from build123d import *

# Parameters (mm, degrees)
SKETCH1_R           = 15
SKETCH1_R_2         = 1.25
SKETCH1_R_3         = 3
BOSS_EXTRUDE1_DEPTH = 5
SKETCH4_R           = 5.5
SKETCH4_R_2         = 5
CUT_EXTRUDE1_DEPTH  = 0.2
SKETCH4_3_R         = 5
SKETCH4_3_R_2       = 3.5
CUT_EXTRUDE2_DEPTH  = 0.1
CUT_EXTRUDE3_START  = -0.1
SKETCH5_R           = 5
SKETCH5_R_2         = 3.5
CUT_EXTRUDE3_DEPTH  = 0.1
CUT_EXTRUDE4_START  = -0.2
SKETCH5_3_R         = 5.75
SKETCH5_3_R_2       = 5
CUT_EXTRUDE4_DEPTH  = 0.2
FILLET1_R           = 0.1


with BuildPart() as part:
    # Sketch1 → Boss-Extrude1 (new body)
    with BuildSketch(Plane(origin=(0, 0, 0), x_dir=(1, 0, 0), z_dir=(0, 1, 0))):
        with Locations(Location((0, 0, 0), (0, 0, 270))):
            Circle(SKETCH1_R)
        with Locations(Location((0, 12, 0), (0, 0, 270))):
            Circle(SKETCH1_R_2, mode=Mode.SUBTRACT)
        with Locations(Location((0, -12, 0), (0, 0, 270))):
            Circle(SKETCH1_R_2, mode=Mode.SUBTRACT)
        with Locations(Location((0, 0, 0), (0, 0, 270))):
            Circle(SKETCH1_R_3, mode=Mode.SUBTRACT)
        with Locations(Location((-12, 0, 0), (0, 0, 270))):
            Circle(SKETCH1_R_2, mode=Mode.SUBTRACT)
        with Locations(Location((12, 0, 0), (0, 0, 270))):
            Circle(SKETCH1_R_2, mode=Mode.SUBTRACT)
        with Locations(Location((8.5, 8.5, 0), (0, 0, 270))):
            Circle(SKETCH1_R_2, mode=Mode.SUBTRACT)
        with Locations(Location((8.5, -8.5, 0), (0, 0, 270))):
            Circle(SKETCH1_R_2, mode=Mode.SUBTRACT)
        with Locations(Location((-8.5, -8.5, 0), (0, 0, 270))):
            Circle(SKETCH1_R_2, mode=Mode.SUBTRACT)
        with Locations(Location((-8.5, 8.5, 0), (0, 0, 270))):
            Circle(SKETCH1_R_2, mode=Mode.SUBTRACT)
    extrude(amount=BOSS_EXTRUDE1_DEPTH)

    # Sketch4 → Cut-Extrude1 (cut)
    with BuildSketch(Plane(origin=(0, 5, 0), x_dir=(1, 0, 0), z_dir=(0, 1, 0))):
        with Locations(Location((0, 0, 0), (0, 0, 270))):
            Circle(SKETCH4_R)
        with Locations(Location((0, 0, 0), (0, 0, 270))):
            Circle(SKETCH4_R_2, mode=Mode.SUBTRACT)
    extrude(amount=-CUT_EXTRUDE1_DEPTH, mode=Mode.SUBTRACT)

    # Sketch4<3> → Cut-Extrude2 (cut)
    with BuildSketch(Plane(origin=(0, 5, 0), x_dir=(1, 0, 0), z_dir=(0, 1, 0))):
        with Locations(Location((0, 0, 0), (0, 0, 270))):
            Circle(SKETCH4_3_R)
        with Locations(Location((0, 0, 0), (0, 0, 270))):
            Circle(SKETCH4_3_R_2, mode=Mode.SUBTRACT)
    extrude(amount=-CUT_EXTRUDE2_DEPTH, mode=Mode.SUBTRACT)

    # Sketch5 → Cut-Extrude3 (cut)
    with BuildSketch(Plane.XZ.offset(CUT_EXTRUDE3_START)):
        with Locations(Location((0, 0, 0), (0, 0, 90))):
            Circle(SKETCH5_R)
        with Locations(Location((0, 0, 0), (0, 0, 90))):
            Circle(SKETCH5_R_2, mode=Mode.SUBTRACT)
    extrude(amount=CUT_EXTRUDE3_DEPTH, mode=Mode.SUBTRACT)

    # Sketch5<3> → Cut-Extrude4 (cut)
    with BuildSketch(Plane.XZ.offset(CUT_EXTRUDE4_START)):
        with Locations(Location((0, 0, 0), (0, 0, 270))):
            Circle(SKETCH5_3_R)
        with Locations(Location((0, 0, 0), (0, 0, 90))):
            Circle(SKETCH5_3_R_2, mode=Mode.SUBTRACT)
    extrude(amount=CUT_EXTRUDE4_DEPTH, mode=Mode.SUBTRACT)

    # Fillet1
    fillet1_edges = [part.edges().sort_by_distance(p)[0] for p in [
        (0, 4.9, -5),
        (0, 0.1, -5),
    ]]
    fillet(fillet1_edges, radius=FILLET1_R - 0.0001)  # a hair under: the kernel refuses the full size


solid = part.part
Check sheet for the modelled part. Datum: model origin and axes. Units: mm. A direction names the side the tool comes from. Give positions to 0.01 mm unless a question says otherwise; leave off trailing zeros. Loops run counter-clockwise (first coordinate to the right, second up) from the corner with the lowest first, then second, coordinate; pieces in that order, holes last. Notation, with made-up numbers: M 58.25,55 L 90.25,55 A13 cw 90.25,69 Z; hole C 56.5,85.5 d8. An arc over 180 degrees is marked long. Return JSON: item names as keys, results as strings. Group by question number.
1. Cross-section at C-C on x = 9. Record the boundary of the cut face in (y, z), plus the area to 3 significant figures.
2. Go/stop test with flat-tipped pins: pin 1 (2 mm diameter, centred on y = 3.5, z = -7, fed in from +X); pin 2 (5.5 mm diameter, centred on x = -1, z = 0.5, fed in from +Y); pin 3 (2 mm diameter, centred on x = 7, y = 2.5, fed in from -Z); pin 4 (1.5 mm diameter, centred on x = 0, z = 12, fed in from +Y). Record where each tip stops, or that it passes through.
3. Cross-section at D-D on z = 8.5. Record the boundary of the cut face in (x, y), plus the area to 3 significant figures.
4. Mould release check, pull along Z, two halves, no side actions. Record for faces 1 (the cylindrical face through (8.55, 2.46, -9.75)), 2 (the flat face through (1, 5, 3)): released by +Z, released by -Z, zero draft, split by the parting line, or undercut.
5. Thickness scan on L1, parallel to X at y = 2.9, z = 0; L2, parallel to X at y = 4.75, z = 0.5; L3, parallel to X at y = 0.15, z = 0. Record the ranges inside material, lowest first.
6. Tool access check on faces 3 (the flat face through (3.2, 0.1, 2.1)), 4 (the flat face through (-3.2, 4.9, 2.1)), 5 (the cylindrical face through (13.24, 2.46, -0.16)). Record the directions out of +Z, -Z, +X, -X, +Y, -Y that give a thin tool (end or side, any length) a straight path to the whole face; none if there is none.
7. Cross-section at B-B on y = 2.65. State how many separate pieces and enclosed holes the cut face has, plus the area to 3 significant figures.
8. Cross-section at A-A on x = 12. Record the boundary of the cut face in (y, z).
Return value:
{
 "1": {"outline": "M 0,-12 L 5,-12 L 5,-9.65 L 0,-9.65 Z; M 0,-7.35 L 5,-7.35 L 5,7.35 L 0,7.35 Z; M 0,9.65 L 5,9.65 L 5,12 L 0,12 Z", "area": "97.1 mm^2"},
 "2": {"pin 1": "x = 13.75", "pin 2": "y = 5", "pin 3": "z = -13.75", "pin 4": "through"},
 "3": {"outline": "M -12.36,0 L -9.75,0 L -9.75,5 L -12.36,5 Z; M -7.25,0 L 7.25,0 L 7.25,5 L -7.25,5 Z; M 9.75,0 L 12.36,0 L 12.36,5 L 9.75,5 Z", "area": "98.6 mm^2"},
 "4": {"face 1": "undercut", "face 2": "zero draft"},
 "5": {"L1": "-15 to -13.25, -10.75 to -3, 3 to 10.75, 13.25 to 15", "L2": "-14.99 to -13.15, -10.85 to -2.96, 2.96 to 10.85, 13.15 to 14.99", "L3": "-15 to -13.25, -10.75 to -5.75, -4.99 to -3, 3 to 4.99, 5.75 to 10.75, 13.25 to 15"},
 "6": {"face 3": "-Y", "face 4": "+Y", "face 5": "+Y, -Y"},
 "7": {"separate pieces": "1", "enclosed holes": "9", "area": "639 mm^2"},
 "8": {"outline": "M 0,-9 L 5,-9 L 5,-1.25 L 0,-1.25 Z; M 0,1.25 L 5,1.25 L 5,9 L 0,9 Z"}
}
